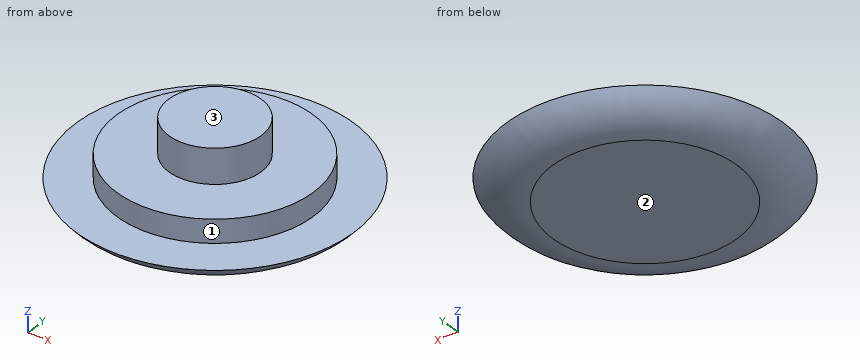
```python
from build123d import *

# Parameters (mm, degrees)
F0_R     = 12
F0_R_2   = 8.5
F1_DEPTH = 2
F0_R_3   = 4
F2_DEPTH = 4
F3_DEPTH = 7


# Not quite as in the source:
# - a fillet or chamfer that OpenCascade refuses, or shapes differently, is made with other operations: its cross-section is extruded or revolved along the edge and cut away or added


with BuildPart() as f1:
    # F0 (on Top) → F1 (new body)
    with BuildSketch(Plane.XY):
        Circle(F0_R)
        Circle(F0_R_2, mode=Mode.SUBTRACT)
    extrude(amount=F1_DEPTH)

    # F0 (on Top) → F2 (join)
    with BuildSketch(Plane.XY):
        Circle(F0_R_2)
        Circle(F0_R_3, mode=Mode.SUBTRACT)
    extrude(amount=F2_DEPTH)

    # F0 (on Top) → F3 (join)
    with BuildSketch(Plane.XY):
        Circle(F0_R_3)
    extrude(amount=F3_DEPTH)

    # F4: fillet of radius 5 on 1 edges, made by hand

    # F4_s1 → F4_t2 (revolve, cut)
    with BuildSketch(Plane.XZ):
        with BuildLine():
            ThreePointArc((12, 2), (10.2360679775, 0.527864045), (8, 0))
            Line((8, 0), (12, 0))
            Line((12, 0), (12, 2))
        make_face()
    revolve(axis=Axis((0, 0, 0), (0, 0, 1)), mode=Mode.SUBTRACT)


solid = f1.part
```
Geometry: final body of the model. Coordinates: model frame, mm. Face numbers are marked on the shaded views. Round coordinates to 2 decimals unless told otherwise and drop trailing zeros. Loops run counter-clockwise (first coordinate to the right, second up) from the corner with the lowest first, then second, coordinate; pieces in that order, holes last.
Item 1: Line query: L1, parallel to Z at x = -3.5, y = 6; L2, parallel to Z at x = 3.5, y = -8.75; L3, parallel to X at y = -6.5, z = 1. Output: solid intervals per line, ascending.
Checked values:
L1: z = 0 to 4
L2: z = 0.21 to 2
L3: x = -8.87 to 8.87
Item 2: Mould query, pull axis Z, two halves, no side actions, for the marked faces 1, 2 and 3. Classes: released by +Z, released by -Z, zero draft, split by the parting line, or undercut.
Checked values:
face 1: zero draft
face 2: released by -Z
face 3: released by +Z
Item 3: Section A-A, the plane x = 0. Output: boundary loops of the cut face in (y, z), plus the area to 3 significant figures.
Checked values:
outline: (-12, 2) arc R5 ccw to (-8, 0) - (8, 0) arc R5 ccw to (12, 2) - (8.5, 2) - (8.5, 4) - (4, 4) - (4, 7) - (-4, 7) - (-4, 4) - (-8.5, 4) - (-8.5, 2) - close
area: 101 mm2
Item 4: Section C-C, the plane z = 1.5. Output: boundary loops of the cut face in (x, y).
Checked values:
outline: circle Ø23.14 at (0, 0)
Item 5: Contact query for flat-ended pins moving along their axis: P1, Ø2, axis at x = -8.5, y = 4.5, coming from the -Z side; P2, Ø8, axis at x = -1, y = 8.5, coming from the +Z side. Output: stop coordinate, or through.
Checked values:
P1: stops at z = 0.04
P2: stops at z = 4
